Read the model definition and answer for the solid it produces. Units are mm, in the model's axes. Face numbers are marked on the shaded views. A direction names the side the tool comes from. Coordinates: 2 decimals unless noted, no trailing zeros. Loops run counter-clockwise (first coordinate to the right, second up) from the corner with the lowest first, then second, coordinate; pieces in that order, holes last.
from build123d import *

# Parameters (mm, degrees)
F0_W     = 60
F0_H     = 16
F1_DEPTH = 10
F2_R     = 2.5
F3_DEPTH = 5
F4_DEPTH = 5


with BuildPart() as f1:
    # F0 (on Top) → F1 (new body)
    with BuildSketch(Plane.XY):
        Rectangle(F0_W, F0_H)
    extrude(amount=F1_DEPTH)

    # F2 (on face) → F3 (join)
    with BuildSketch(Plane.XY.offset(10)):
        Circle(F2_R)
    extrude(amount=F3_DEPTH)

    # F2 (on face) → F4 (join)
    with BuildSketch(Plane.XY.offset(10)):
        with Locations((-20, 0)):
            Circle(F2_R)
        Circle(F2_R)
    extrude(amount=F4_DEPTH)


solid = f1.part
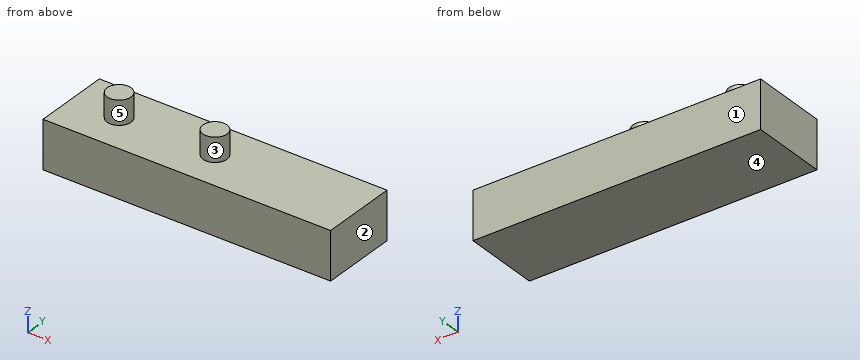
Item 1: A cutting plane is placed at B-B on y = 0. Determine the outline of the cut face in (x, z), then the cut area to 3 significant figures.
Numbers:
outline: (-30, 0) - (30, 0) - (30, 10) - (2.5, 10) - (2.5, 15) - (-2.5, 15) - (-2.5, 10) - (-17.5, 10) - (-17.5, 15) - (-22.5, 15) - (-22.5, 10) - (-30, 10) - close
area: 650 mm2
Item 2: Given pin 1 (5 mm diameter, centred on x = -4.5, y = -4, fed in from +Z), flat-ended and moving along its own axis, determine where the tip first touches the part or whether it passes through.
Numbers:
pin 1: stops at z = 10
Item 3: A cutting plane is placed at A-A on x = 0. Determine the outline of the cut face in (y, z), then the cut area to 3 significant figures.
Numbers:
outline: (-8, 0) - (8, 0) - (8, 10) - (2.5, 10) - (2.5, 15) - (-2.5, 15) - (-2.5, 10) - (-8, 10) - close
area: 185 mm2
Item 4: A cutting plane is placed at C-C on x = -21. Determine the outline of the cut face in (y, z), then the cut area to 3 significant figures.
Numbers:
outline: (-8, 0) - (8, 0) - (8, 10) - (2.29, 10) - (2.29, 15) - (-2.29, 15) - (-2.29, 10) - (-8, 10) - close
area: 183 mm2
Item 5: A cutting plane is placed at D-D on y = 4.5. Determine the outline of the cut face in (x, z), then the cut area to 3 significant figures.
Numbers:
outline: (-30, 0) - (30, 0) - (30, 10) - (-30, 10) - close
area: 600 mm2
Item 6: Determine the mould class of the marked faces 1, 2 and 3 for opening direction X: released by +X, released by -X, zero draft, split by the parting line, or undercut.
Numbers:
face 1: zero draft
face 2: released by +X
face 3: undercut
Item 7: Which of the six approach directions +Z, -Z, +X, -X, +Y, -Y give full straight-line access (tool end or side, diameter ignored) to the marked faces 4 and 5?
Numbers:
face 4: -Z, +X, -X, +Y, -Y
face 5: +Z
Item 8: Find the intervals of material crossed by line 1 along Z through (x, y) = (-23.5, 3), in increasing order.
Numbers:
line 1: z = 0 to 10
